Source: CAD feature listing. Evaluate the final solid. Frame: model axes, mm. A direction names the side the tool comes from. Round coordinates to 2 decimals unless told otherwise and drop trailing zeros. Loops run counter-clockwise (first coordinate to the right, second up) from the corner with the lowest first, then second, coordinate; pieces in that order, holes last. Notation, with made-up numbers: (40, 12) - (90, 12) arc R27 ccw to (90, 40) - close; hole circle Ø10 at (66.25, -2). An arc over 180 degrees is marked (long way). One line per question, with ' | ' between items.
from build123d import *

# Parameters (mm, degrees)
F0_W      = 14.732
F0_H      = 1.1938
F1_DEPTH  = 0.889
F2_W      = 1.1938
F2_H      = 24.892
F3_DEPTH  = 1.4986
F4_R      = 0.381
F5_DEPTH  = 1.1938
F6_R      = 0.381
F7_DEPTH  = 1.1938
F8_R      = 0.508
F9_W      = 3.048
F9_H      = 1.1938
F10_DEPTH = 0.889
F11_W     = 1.016
F11_H     = 1.1938
F12_DEPTH = 2.3876
F13_W     = 4.572
F13_H     = 1.4986
F14_DEPTH = 1.016


with BuildPart() as f1:
    # F0 (on Top) → F1 (new body)
    with BuildSketch(Plane.XY):
        with Locations((0, 9.8171)):
            Rectangle(F0_W, F0_H)
    extrude(amount=F1_DEPTH)



with BuildPart() as f1b:
    # F0 (on Top) → F1, piece 2 (new body)
    with BuildSketch(Plane.XY):
        with Locations((0, -9.8171)):
            Rectangle(F0_W, F0_H)
    extrude(amount=F1_DEPTH)


with BuildPart() as f1c:
    # F0 (on Top) → F1, piece 3 (new body)
    with BuildSketch(Plane.XY):
        with Locations((0, -5.5753)):
            Rectangle(F0_W, F0_H)
    extrude(amount=F1_DEPTH)


with BuildPart() as f1d:
    # F0 (on Top) → F1, piece 4 (new body)
    with BuildSketch(Plane.XY):
        Rectangle(F0_W, F0_H)
    extrude(amount=F1_DEPTH)


with BuildPart() as f1e:
    # F0 (on Top) → F1, piece 5 (new body)
    with BuildSketch(Plane.XY):
        with Locations((0, 5.5753)):
            Rectangle(F0_W, F0_H)
    extrude(amount=F1_DEPTH)


with BuildPart() as f1_1:
    add(f1.part)

    add(f1b.part)  # F3 merges F1b

    add(f1c.part)  # F3 merges F1c

    add(f1d.part)  # F3 merges F1d

    add(f1e.part)  # F3 merges F1e
    # F2 (on face) → F3 (join)
    with BuildSketch(Plane.XY.offset(0.889)):
        with Locations((-6.7691, 0)):
            Rectangle(F2_W, F2_H)
        with Locations((6.7691, 0)):
            Rectangle(F2_W, F2_H)
        with Locations((-1.6129, 0)):
            Rectangle(F2_W, F2_H)
        with Locations((1.6129, 0)):
            Rectangle(F2_W, F2_H)
    extrude(amount=F3_DEPTH)

    # F4 (on face) → F5 (join)
    with BuildSketch(Plane(origin=(-7.366, 0, 0), x_dir=(0, -1, 0), z_dir=(-1, 0, 0))):
        Polygon((-6.604, 4.2545157337), (-7.874, 2.3876), (-3.302, 2.3876), (-4.572, 4.2545157337), align=None)
        with Locations((-5.588, 3.2385157337)):
            Circle(F4_R, mode=Mode.SUBTRACT)
        Polygon((4.572, 4.2545157337), (3.302, 2.3876), (7.874, 2.3876), (6.604, 4.2545157337), align=None)
        with Locations((5.588, 3.2385157337)):
            Circle(F4_R, mode=Mode.SUBTRACT)
    extrude(amount=-F5_DEPTH)

    # F6 (on face) → F7 (join)
    with BuildSketch(Plane.YZ.offset(7.366)):
        Polygon((-6.604, 4.2545157337), (-7.874, 2.3876), (-3.302, 2.3876), (-4.572, 4.2545157337), align=None)
        with Locations((-5.588, 3.2385157337)):
            Circle(F6_R, mode=Mode.SUBTRACT)
        Polygon((3.302, 2.3876), (7.874, 2.3876), (6.604, 4.2545157337), (4.572, 4.2545157337), align=None)
        with Locations((5.588, 3.2385157337)):
            Circle(F6_R, mode=Mode.SUBTRACT)
    extrude(amount=-F7_DEPTH)

    # F8
    f8_edges = [f1_1.edges().sort_by_distance(p)[0] for p in [
        (6.7691, -4.572, 4.254516),
        (6.7691, -6.604, 4.254516),
        (6.7691, -3.302, 2.3876),
        (6.7691, -7.874, 2.3876),
        (6.7691, 4.572, 4.254516),
        (6.7691, 3.302, 2.3876),
        (6.7691, 6.604, 4.254516),
        (6.7691, 7.874, 2.3876),
        (-6.7691, 7.874, 2.3876),
        (-6.7691, 6.604, 4.254516),
        (-6.7691, 4.572, 4.254516),
        (-6.7691, 3.302, 2.3876),
        (-6.7691, -7.874, 2.3876),
        (-6.7691, -6.604, 4.254516),
        (-6.7691, -4.572, 4.254516),
        (-6.7691, -3.302, 2.3876),
    ]]
    fillet(f8_edges, radius=F8_R)

    # F9 (on face) → F10 (cut, through all)
    with BuildSketch(Plane(origin=(0, 0, 0), x_dir=(1, 0, 0), z_dir=(0, 0, -1))):
        Rectangle(F9_W, F9_H)
    extrude(amount=-F10_DEPTH, mode=Mode.SUBTRACT)

    # F11 (on face) → F12 (join, through all)
    with BuildSketch(Plane(origin=(0, 0, 0), x_dir=(1, 0, 0), z_dir=(0, 0, -1))):
        with Locations((7.874, 0)):
            Rectangle(F11_W, F11_H)
    extrude(amount=-F12_DEPTH)

    # F13 (on face) → F14 (join, through all)
    with BuildSketch(Plane.YZ.offset(8.382)):
        with Locations((0, 1.6383)):
            Rectangle(F13_W, F13_H)
    extrude(amount=-F14_DEPTH)


solid = f1_1.part
1. Section query D-D, the plane x = 4.5. Return loops of the section in (y, z), plus the area to 3 significant figures.
Worked out:
outline: (-10.41, 0) - (-9.22, 0) - (-9.22, 0.89) - (-10.41, 0.89) - close; (-6.17, 0) - (-4.98, 0) - (-4.98, 0.89) - (-6.17, 0.89) - close; (-0.6, 0) - (0.6, 0) - (0.6, 0.89) - (-0.6, 0.89) - close; (4.98, 0) - (6.17, 0) - (6.17, 0.89) - (4.98, 0.89) - close; (9.22, 0) - (10.41, 0) - (10.41, 0.89) - (9.22, 0.89) - close | area: 5.31 mm2
2. Material intervals for probe 1 along X at (y, z) = (7, 1.95); probe 2 along Y at (x, z) = (-1, 0.7); probe 3 along Y at (x, z) = (3.5, 0.75), sorted ascending.
Worked out:
probe 1: x = -7.37 to -6.17, -2.21 to -1.02, 1.02 to 2.21, 6.17 to 7.37 | probe 2: y = -10.41 to -9.22, -6.17 to -4.98, 4.98 to 6.17, 9.22 to 10.41 | probe 3: y = -10.41 to -9.22, -6.17 to -4.98, -0.6 to 0.6, 4.98 to 6.17, 9.22 to 10.41
3. Contact query for flat-ended pins moving along their axis: P1, Ø0.7, axis at x = -4.5, z = 0.5, coming from the -Y side; P2, Ø0.6, axis at x = 4.5, y = -6, coming from the +Z side; P3, Ø0.6, axis at x = -2, y = -11.5, coming from the -Z side. Output: stop coordinate, or through.
Worked out:
P1: stops at y = -10.41 | P2: stops at z = 0.89 | P3: stops at z = 0.89
4. Section query C-C, the plane x = 0.5. Return loops of the section in (y, z), plus the area to 3 significant figures.
Worked out:
outline: (-10.41, 0) - (-9.22, 0) - (-9.22, 0.89) - (-10.41, 0.89) - close; (-6.17, 0) - (-4.98, 0) - (-4.98, 0.89) - (-6.17, 0.89) - close; (4.98, 0) - (6.17, 0) - (6.17, 0.89) - (4.98, 0.89) - close; (9.22, 0) - (10.41, 0) - (10.41, 0.89) - (9.22, 0.89) - close | area: 4.25 mm2
5. Access query for faces 5 (the flat face through (-2, 11, 0.889)), 6 (the flat face through (4, 10, 0.889)), 7 (the flat face through (2, -11, 0.889)), 8 (the flat face through (7, -2, 0.889)), 9 (the flat face through (-6.78, 3.93, 3.31)). Directions: +Z, -Z, +X, -X, +Y, -Y. A direction counts if a zero-diameter tool reaches every point of the face in a straight line with its end or side. Return the directions, or none.
Worked out:
face 5: -Z, +X, -X, +Y | face 6: +Z, +Y, -Y | face 7: -Z, +X, -X, -Y | face 8: -Z, +X, -X | face 9: +Z, +X, -X
6. Section query B-B, the plane z = 2.1. Return loops of the section in (x, y), plus the area to 3 significant figures.
Worked out:
outline: (-7.37, -12.45) - (-6.17, -12.45) - (-6.17, 12.45) - (-7.37, 12.45) - close; (-2.21, -12.45) - (-1.02, -12.45) - (-1.02, 12.45) - (-2.21, 12.45) - close; (1.02, -12.45) - (2.21, -12.45) - (2.21, 12.45) - (1.02, 12.45) - close; (6.17, -12.45) - (7.37, -12.45) - (7.37, -2.29) - (8.38, -2.29) - (8.38, 2.29) - (7.37, 2.29) - (7.37, 12.45) - (6.17, 12.45) - close | area: 124 mm2
7. Mould query, pull axis Y, two halves, no side actions, for faces 1 (the flat face through (7.366, -7, 2)), 2 (the flat face through (-0.1, -10.414, 0.4)), 3 (the flat face through (-0.1, -9.22, 0.4)), 4 (the flat face through (1.3, 0.1, 0.889)). Classes: released by +Y, released by -Y, zero draft, split by the parting line, or undercut.
Worked out:
face 1: zero draft | face 2: released by -Y | face 3: undercut | face 4: undercut
8. Section query A-A, the plane y = -2. Return loops of the section in (x, z), plus the area to 3 significant figures.
Worked out:
outline: (-7.37, 0.89) - (-6.17, 0.89) - (-6.17, 2.39) - (-7.37, 2.39) - close; (-2.21, 0.89) - (-1.02, 0.89) - (-1.02, 2.39) - (-2.21, 2.39) - close; (1.02, 0.89) - (2.21, 0.89) - (2.21, 2.39) - (1.02, 2.39) - close; (6.17, 0.89) - (8.38, 0.89) - (8.38, 2.39) - (6.17, 2.39) - close | area: 8.68 mm2
